Verification items for the finished model (mm, model axes). A direction names the side the tool comes from. Coordinates: 2 decimals unless noted, no trailing zeros. Loops run counter-clockwise (first coordinate to the right, second up) from the corner with the lowest first, then second, coordinate; pieces in that order, holes last. Notation, with made-up numbers: (72.25, -12.75) - (125.25, -12.75) arc R20 cw to (125.25, 7.25) - close; hole circle Ø2 at (48.5, 85). An arc over 180 degrees is marked (long way). One line per item, written item: value. Start each with the question number.
(1) Section check B-B (x = -246). Record the boundary of the cut face in (y, z).
(2) Section check C-C (z = -189.5). Record the boundary of the cut face in (x, y), plus the area to 3 significant figures.
(3) Section check D-D (z = -66). Record the boundary of the cut face in (x, y).
(4) Gauge pin test, flat ends, axial feed: P1, Ø9.5, axis at x = -257, y = 13.5, coming from the +Z side; P2, Ø8, axis at y = 13.5, z = -164.5, coming from the +X side; P3, Ø9.5, axis at x = -69.5, y = 17, coming from the +Z side; P4, Ø13, axis at y = 11.5, z = -249.5, coming from the -X side. Record the tip position at first contact, or that the pin passes through.
(5) Set-up check for faces 1 (the face through (-77, 14, -142.664)), 2 (the face through (-3, 13, -152.664)), 3 (the face through (-152, 20, -153)): record each of +Z, -Z, +X, -X, +Y, -Y from which the full face is reachable in a straight line by a thin tool's end or side.
(6) Thickness scan on probe 1 along Y at (x, z) = (-52.5, -40); probe 2 along Z at (x, y) = (-105, 13.5); probe 3 along Z at (x, y) = (-73, 14.5). Record the ranges inside material, lowest first. Write a range as [from, to].
(7) Draft check along X on faces 4 (the face through (-143, 60, -13)), 5 (the face through (-142.664, 14, -229)), 6 (the face through (-260.051, 45.192, -251.135)), 7 (the face through (0, 13, -75)). Enter one of: +X half, -X half, draft (parallel to the pull), parting line (faces both ways), or undercut.
(8) Section check A-A (y = 33). Record the boundary of the cut face in (x, z), plus the area to 3 significant figures.
```python
from build123d import *

# Parameters (mm, degrees)
SKETCH1_R           = 145.7
SKETCH1_R_2         = 139.7
BOSS_EXTRUDE1_DEPTH = 60
SKETCH2_R           = 15
BOSS_EXTRUDE2_DEPTH = 12
BOSS_EXTRUDE3_DEPTH = 10
SKETCH4_R           = 1.5
CUT_EXTRUDE1_DEPTH  = 62
SKETCH1_2_R         = 145.7
SKETCH1_2_R_2       = 139.7
CUT_EXTRUDE2_DEPTH  = 8
SKETCH5_W           = 20
SKETCH5_H           = 120
CUT_EXTRUDE3_DEPTH  = 55
CIRPATTERN1_COUNT   = 4
SKETCH6_R           = 1.5
CUT_EXTRUDE4_DEPTH  = 37


with BuildPart() as part:
    # Sketch1 → Boss-Extrude1 (new body)
    with BuildSketch(Plane(origin=(0, 0, 0), x_dir=(1, 0, 0), z_dir=(0, 1, 0))):
        with Locations((-152.664354058, 152.664354058)):
            Circle(SKETCH1_R)
        with Locations((-152.664354058, 152.664354058)):
            Circle(SKETCH1_R_2, mode=Mode.SUBTRACT)
    extrude(amount=BOSS_EXTRUDE1_DEPTH)

    # Sketch2 → Boss-Extrude2 (add)
    with BuildSketch(Plane(origin=(0, 8, 0), x_dir=(-1, 0, 0), z_dir=(0, -1, 0))):
        with BuildLine():
            ThreePointArc((13.322723524, 162.664354058), (12.964354058, 152.664354058), (13.322723524, 142.664354058))
            Line((13.322723524, 142.664354058), (137.664354058, 142.664354058))
            Line((137.664354058, 142.664354058), (141.484014171, 142.664354058))
            ThreePointArc((141.484014171, 142.664354058), (137.664354058, 152.664354058), (141.484014171, 162.664354058))
            Line((141.484014171, 162.664354058), (137.664354058, 162.664354058))
            Line((137.664354058, 162.664354058), (13.322723524, 162.664354058))
        make_face()
        with BuildLine():
            ThreePointArc((162.664354058, 292.005984593), (152.664354058, 292.364354058), (142.664354058, 292.005984593))
            Line((142.664354058, 292.005984593), (142.664354058, 167.664354058))
            Line((142.664354058, 167.664354058), (142.664354058, 163.844693946))
            ThreePointArc((142.664354058, 163.844693946), (152.664354058, 167.664354058), (162.664354058, 163.844693946))
            Line((162.664354058, 163.844693946), (162.664354058, 167.664354058))
            Line((162.664354058, 167.664354058), (162.664354058, 292.005984593))
        make_face()
        with BuildLine():
            Line((167.664354058, 142.664354058), (292.005984593, 142.664354058))
            ThreePointArc((292.005984593, 142.664354058), (292.274732945, 147.661144372), (292.364354058, 152.664354058))
            ThreePointArc((292.364354058, 152.664354058), (292.274732945, 157.667563745), (292.005984593, 162.664354058))
            Line((292.005984593, 162.664354058), (167.664354058, 162.664354058))
            Line((167.664354058, 162.664354058), (163.844693946, 162.664354058))
            ThreePointArc((163.844693946, 162.664354058), (166.676939443, 158.016685405), (167.664354058, 152.664354058))
            ThreePointArc((167.664354058, 152.664354058), (166.676939443, 147.312022712), (163.844693946, 142.664354058))
            Line((163.844693946, 142.664354058), (167.664354058, 142.664354058))
        make_face()
        with BuildLine():
            Line((142.664354058, 141.484014171), (142.664354058, 137.664354058))
            Line((142.664354058, 137.664354058), (142.664354058, 13.322723524))
            ThreePointArc((142.664354058, 13.322723524), (152.664354058, 12.964354058), (162.664354058, 13.322723524))
            Line((162.664354058, 13.322723524), (162.664354058, 137.664354058))
            Line((162.664354058, 137.664354058), (162.664354058, 141.484014171))
            ThreePointArc((162.664354058, 141.484014171), (152.664354058, 137.664354058), (142.664354058, 141.484014171))
        make_face()
        with Locations((152.664354058, 152.664354058)):
            Circle(SKETCH2_R)
    extrude(amount=-BOSS_EXTRUDE2_DEPTH)

    # Sketch3 → Boss-Extrude3 (add)
    with BuildSketch(Plane(origin=(0, 8, 0), x_dir=(-1, 0, 0), z_dir=(0, -1, 0))):
        with BuildLine():
            Line((152.664354058, 6.964354058), (152.664354058, 0))
            Line((152.664354058, 0), (0, 0))
            Line((0, 0), (0, 152.664354058))
            Line((0, 152.664354058), (6.964354058, 152.664354058))
            ThreePointArc((6.964354058, 152.664354058), (49.638896039, 49.638896039), (152.664354058, 6.964354058))
        make_face()
    extrude(amount=-BOSS_EXTRUDE3_DEPTH)

    # Sketch4 → Cut-Extrude1 (cut)
    with BuildSketch(Plane(origin=(0, 18, 0), x_dir=(1, 0, 0), z_dir=(0, 1, 0))):
        with Locations((-122.664354058, 3.482177029)):
            Circle(SKETCH4_R)
        with Locations((-20, 3.482177029)):
            Circle(SKETCH4_R)
        with Locations((-20, 20.002177029)):
            Circle(SKETCH4_R)
        with Locations((-3.482177029, 20.002177029)):
            Circle(SKETCH4_R)
        with Locations((-3.482177029, 3.482177029)):
            Circle(SKETCH4_R)
        with Locations((-3.482177029, 122.664354058)):
            Circle(SKETCH4_R)
    extrude(amount=-CUT_EXTRUDE1_DEPTH, mode=Mode.SUBTRACT)

    # Sketch1<2> → Cut-Extrude2 (cut)
    with BuildSketch(Plane(origin=(0, 0, 0), x_dir=(1, 0, 0), z_dir=(0, 1, 0))):
        with Locations((-152.664354058, 152.664354058)):
            Circle(SKETCH1_2_R)
        with Locations((-152.664354058, 152.664354058)):
            Circle(SKETCH1_2_R_2, mode=Mode.SUBTRACT)
    extrude(amount=CUT_EXTRUDE2_DEPTH, mode=Mode.SUBTRACT)

    # Sketch5 → Cut-Extrude3 (cut)
    with BuildSketch(Plane(origin=(-255.689812077, 0, -255.689812077), x_dir=(0, -1, 0), z_dir=(-0.707106781, 0, -0.707106781))):
        with Locations((-34, 0)):
            Rectangle(SKETCH5_W, SKETCH5_H)
    cut_extrude3 = extrude(amount=-CUT_EXTRUDE3_DEPTH, mode=Mode.SUBTRACT)

    # CirPattern1: Cut-Extrude3 ×4 about axis
    cirpattern1_axis = Axis((-152.664354058, 0, -152.664354058), (0, 1, 0))
    for i in range(1, CIRPATTERN1_COUNT):
        add(cut_extrude3.rotate(cirpattern1_axis, i * 360 / CIRPATTERN1_COUNT), mode=Mode.SUBTRACT)

    # Sketch6 → Cut-Extrude4 (cut)
    with BuildSketch(Plane(origin=(0, 20, 0), x_dir=(1, 0, 0), z_dir=(0, 1, 0))):
        with BuildLine():
            ThreePointArc((-144.104525473, 148.543755244), (-146.092112388, 148.103034136), (-145.809681622, 146.086857134))
            ThreePointArc((-145.809681622, 146.086857134), (-143.627521762, 146.392539165), (-144.104525473, 148.543755244))
        make_face()
        with Locations((-157.22567398, 146.092112388)):
            Circle(SKETCH6_R)
        with Locations((-148.103034136, 159.236595728)):
            Circle(SKETCH6_R)
        with BuildLine():
            ThreePointArc((-159.519026494, 159.241850983), (-161.701186354, 158.936168951), (-161.224182644, 156.784952872))
            ThreePointArc((-161.224182644, 156.784952872), (-159.236595728, 157.22567398), (-159.519026494, 159.241850983))
        make_face()
    extrude(amount=-CUT_EXTRUDE4_DEPTH, mode=Mode.SUBTRACT)


solid = part.part
```
Responses:
1. outline: (8, -264.54) - (24, -264.54) - (24, -256.61) - (8, -256.61) - close; (8, -162.66) - (20, -162.66) - (20, -142.66) - (8, -142.66) - close; (8, -48.72) - (24, -48.72) - (24, -40.79) - (8, -40.79) - close; (44, -264.54) - (60, -264.54) - (60, -256.61) - (44, -256.61) - close; (44, -48.72) - (60, -48.72) - (60, -40.79) - (44, -40.79) - close
2. outline: (-293.63, 8) - (-287.42, 8) - (-287.42, 60) - (-293.63, 60) - close; (-162.66, 8) - (-142.66, 8) - (-142.66, 20) - (-162.66, 20) - close; (-17.91, 8) - (-11.7, 8) - (-11.7, 60) - (-17.91, 60) - close
2. area: 886 mm²
3. outline: (-269.79, 8) - (-262.23, 8) - (-262.23, 24) - (-269.79, 24) - close; (-269.79, 44) - (-262.23, 44) - (-262.23, 60) - (-269.79, 60) - close; (-162.66, 8) - (-142.66, 8) - (-142.66, 20) - (-162.66, 20) - close; (-43.1, 8) - (0, 8) - (0, 18) - (-35.54, 18) - (-35.54, 24) - (-43.1, 24) - close; (-43.1, 44) - (-35.54, 44) - (-35.54, 60) - (-43.1, 60) - close
4. P1: stops at z = -46.31
4. P2: stops at x = -7.18
4. P3: stops at z = 0
4. P4: stops at x = -266.98
5. face 1: +Y, -Y
5. face 2: -Z, +X, +Y, -Y
5. face 3: +Y
6. probe 1: y = [8, 18]
6. probe 2: z = [-290.35, -283.98], [-162.66, -142.66], [-21.35, 0]
6. probe 3: z = [-274.66, -267.42], [-162.66, -142.66], [-37.91, 0]
7. face 4: draft
7. face 5: undercut
7. face 6: parting line
7. face 7: +X half
8. outline: (-288.97, -204.12) - (-284.3, -199.45) arc R139.7 cw to (-284.3, -105.88) - (-288.97, -101.21) arc R145.7 ccw to start; (-204.12, -288.97) arc R145.7 ccw to (-101.21, -288.97) - (-105.88, -284.3) arc R139.7 cw to (-199.45, -284.3) - close; (-204.12, -16.35) - (-199.45, -21.03) arc R139.7 cw to (-105.88, -21.03) - (-101.21, -16.35) arc R145.7 ccw to start; (-21.03, -199.45) - (-16.35, -204.12) arc R145.7 ccw to (-16.35, -101.21) - (-21.03, -105.88) arc R139.7 cw to start
8. area: 2,410 mm²
